Geometry check sheet. Reference: the model listing, model coordinates, mm. Face numbers are marked on the shaded views. A direction names the side the tool comes from. Coordinates: 2 decimals unless noted, no trailing zeros. Loops run counter-clockwise (first coordinate to the right, second up) from the corner with the lowest first, then second, coordinate; pieces in that order, holes last.
from build123d import *

# Parameters (mm, degrees)
BOSS_EXTRUDE1_DEPTH = 6.1722
SKETCH3_R           = 2.4511
BOSS_EXTRUDE2_DEPTH = 4.8895


with BuildPart() as part:
    # Sketch2 → Boss-Extrude1 (new body)
    with BuildSketch(Plane(origin=(0, 0, 0), x_dir=(1, 0, 0), z_dir=(0, 1, 0))):
        with BuildLine():
            Line((-1.968459032, 1.4605), (1.968459032, 1.4605))
            ThreePointArc((1.968459032, 1.4605), (2.4511, 0), (1.968459032, -1.4605))
            Line((1.968459032, -1.4605), (-1.968459032, -1.4605))
            ThreePointArc((-1.968459032, -1.4605), (-2.4511, 0), (-1.968459032, 1.4605))
        make_face()
    extrude(amount=-BOSS_EXTRUDE1_DEPTH)

    # Sketch3 → Boss-Extrude2 (add)
    with BuildSketch(Plane.XZ.offset(6.1722)):
        Circle(SKETCH3_R)
    extrude(amount=BOSS_EXTRUDE2_DEPTH)


solid = part.part
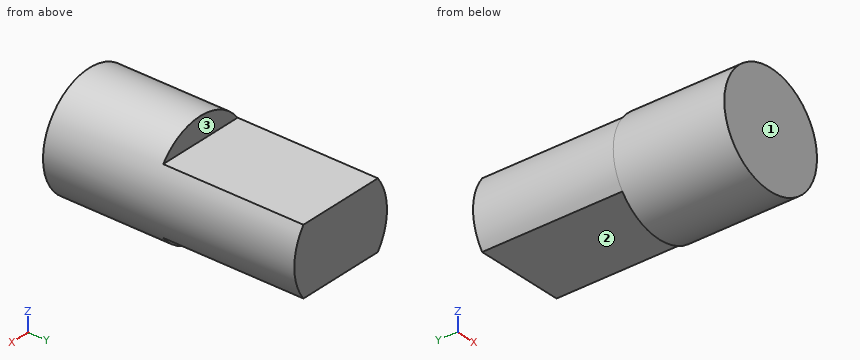
1) Material ranges on probe 1 along Z at (x, y) = (-1.5, -3.5); probe 2 along Y at (x, z) = (-0.9, -1.7); probe 3 along Z at (x, y) = (-1.05, -10.5), recorded low to high.
Data:
probe 1: z = -1.46 to 1.46
probe 2: y = -11.06 to -6.17
probe 3: z = -2.21 to 2.21
2) Access from +Z, -Z, +X, -X, +Y, -Y to the whole of each face (thin tool, end or side, straight path). Record for the marked faces 1, 2 and 3.
Data:
face 1: +Z, -Z, +X, -X, -Y
face 2: -Z, +X, -X, +Y
face 3: +Z, +X, -X, +Y
3) Section check B-B on y = -3. Record the cut outline in (x, z).
Data:
outline: (-1.97, -1.46) - (1.97, -1.46) arc R2.45 ccw to (1.97, 1.46) - (-1.97, 1.46) arc R2.45 ccw to start
4) Section check A-A on x = 0. Record the cut outline in (y, z).
Data:
outline: (-11.06, -2.45) - (-6.17, -2.45) - (-6.17, -1.46) - (0, -1.46) - (0, 1.46) - (-6.17, 1.46) - (-6.17, 2.45) - (-11.06, 2.45) - close
5) Depth check by flat-ended pin: pin 1 (1 mm diameter, centred on x = 1.5, y = -8.5, fed in from -Z); pin 2 (2 mm diameter, centred on x = 0.5, z = -1.5, fed in from +Y); pin 3 (1.2 mm diameter, centred on x = 0, y = -4.5, fed in from +Z); pin 4 (0.5 mm diameter, centred on x = 0.5, z = -2, fed in from +Y). Enter the tip coordinate at first touch or a pass-through.
Data:
pin 1: stops at z = -2.24
pin 2: stops at y = 0
pin 3: stops at z = 1.46
pin 4: stops at y = -6.17
6) Section check D-D on x = -1. Record the cut outline in (y, z), and give its area (3 significant figures).
Data:
outline: (-11.06, -2.24) - (-6.17, -2.24) - (-6.17, -1.46) - (0, -1.46) - (0, 1.46) - (-6.17, 1.46) - (-6.17, 2.24) - (-11.06, 2.24) - close
area: 39.9 mm2
7) Section check C-C on z = 1.8. Record the cut outline in (x, y).
Data:
outline: (-1.66, -11.06) - (1.66, -11.06) - (1.66, -6.17) - (-1.66, -6.17) - close
